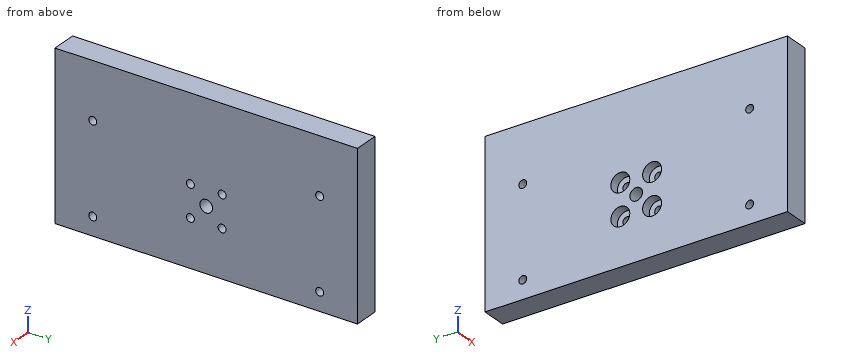
from build123d import *

# Parameters (mm, degrees)
ESQUISSE1_W             = 82.55
ESQUISSE1_H             = 152.4
BOSS_EXTRU_1_DEPTH      = 12.7
ESQUISSE2_R             = 2
ENL_V_MAT_EXTRU_1_DEPTH = 88.586275323
ESQUISSE3_R             = 3.175
ESQUISSE3_R_2           = 2
ENL_V_MAT_EXTRU_2_DEPTH = 88.586275323
ESQUISSE4_R             = 4.7625
ENL_V_MAT_EXTRU_3_DEPTH = 4.7625


with BuildPart() as part:
    # Esquisse1 → Boss.-Extru.1 (new body)
    with BuildSketch(Plane(origin=(0, 0, 0), x_dir=(0, 0, -1), z_dir=(1, 0, 0))):
        Rectangle(ESQUISSE1_W, ESQUISSE1_H)
    extrude(amount=BOSS_EXTRU_1_DEPTH)

    # Esquisse2 → Enlèv. mat.-Extru.1 (cut, through all)
    with BuildSketch(Plane(origin=(12.7, 0, 0), x_dir=(0, 0, -1), z_dir=(1, 0, 0))):
        with Locations((-12.974999958, 57.15)):
            Circle(ESQUISSE2_R)
        with Locations((32.025000042, 57.15)):
            Circle(ESQUISSE2_R)
        with Locations((-12.974999958, -57.15)):
            Circle(ESQUISSE2_R)
        with Locations((32.025000042, -57.15)):
            Circle(ESQUISSE2_R)
    extrude(amount=-ENL_V_MAT_EXTRU_1_DEPTH, mode=Mode.SUBTRACT)

    # Esquisse3 → Enlèv. mat.-Extru.2 (cut, through all)
    with BuildSketch(Plane(origin=(12.7, 0, 0), x_dir=(0, 0, -1), z_dir=(1, 0, 0))):
        with Locations((9.525, 0)):
            Circle(ESQUISSE3_R)
        with Locations((17.525, 8)):
            Circle(ESQUISSE3_R_2)
        with Locations((1.525, 8)):
            Circle(ESQUISSE3_R_2)
        with Locations((1.525, -8)):
            Circle(ESQUISSE3_R_2)
        with Locations((17.525, -8)):
            Circle(ESQUISSE3_R_2)
    extrude(amount=-ENL_V_MAT_EXTRU_2_DEPTH, mode=Mode.SUBTRACT)

    # Esquisse4 → Enlèv. mat.-Extru.3 (cut)
    with BuildSketch(Plane(origin=(0, 0, 0), x_dir=(0, 0, -1), z_dir=(1, 0, 0))):
        with Locations(Location((17.525, 8, 0), (0, 0, 180))):
            Circle(ESQUISSE4_R)
        with Locations(Location((1.525, 8, 0), (0, 0, 180))):
            Circle(ESQUISSE4_R)
        with Locations(Location((1.525, -8, 0), (0, 0, 180))):
            Circle(ESQUISSE4_R)
        with Locations(Location((17.525, -8, 0), (0, 0, 180))):
            Circle(ESQUISSE4_R)
    extrude(amount=ENL_V_MAT_EXTRU_3_DEPTH, mode=Mode.SUBTRACT)


solid = part.part
Build history of the part. All positions in model axes, mm. Coordinates: 2 decimals unless noted, no trailing zeros. Write each loop counter-clockwise with the first axis right and the second up, starting at its lowest first coordinate (ties: lowest second). Pieces come first, ordered by that corner, then holes. Notation, with made-up numbers: (-3.5, 53.25) -> (13.5, 53.25) arc R12 ccw to (13.5, 73.25) -> close; hole circle Ø1 at (70.5, 58). An arc over 180 degrees is marked (long way). Use CSV: the item, a comma, the result in double quotes. Start each with the question number.
Q1. Cut at A-A, the plane y = 8. List the corners of the cut face in (x, z) (1 decimal), then the cut area to 3 significant figures.
Q2. Drill centre lines: probe 1 along Y at (x, z) = (7.5, -31); probe 2 along Z at (x, y) = (1.25, 11) (3 decimals); probe 3 along Z at (x, y) = (7.5, 58) (3 decimals). Where is each one in solid material? Low to high.
Q3. Cut at B-B, the plane x = 3. State how many separate pieces and enclosed holes the cut face has, then the cut area to 3 significant figures.
Q4. Cut at C-C, the plane y = 57.15. List the corners of the cut face in (x, z) (3 decimals), then the cut area to 3 significant figures.
Q5. Flat gauge pins, fed straight in: pin 1 Ø3 at (y, z) = (9, -1.5) entering from -X; pin 2 Ø7.5 at (y, z) = (-8, -17.525) entering from +X. Where does each tip first touch, or does it go through?
Checked values:
1,outline,"(0, -41.3) -> (12.7, -41.3) -> (12.7, -19.5) -> (4.8, -19.5) -> (4.8, -22.3) -> (0, -22.3) -> close; (0, -12.8) -> (4.8, -12.8) -> (4.8, -15.5) -> (12.7, -15.5) -> (12.7, -3.5) -> (4.8, -3.5) -> (4.8, -6.3) -> (0, -6.3) -> close; (0, 3.2) -> (4.8, 3.2) -> (4.8, 0.5) -> (12.7, 0.5) -> (12.7, 41.3) -> (0, 41.3) -> close"
1,area,"894 mm²"
2,probe 1,"y = -76.2 to -58.87, -55.43 to 55.43, 58.87 to 76.2"
2,probe 2,"z = -41.275 to -21.224, -13.826 to -5.224, 2.174 to 41.275"
2,probe 3,"z = -41.275 to -33.835, -30.215 to 11.165, 14.785 to 41.275"
3,separate pieces,"1"
3,enclosed holes,"9"
3,area,"12,200 mm²"
4,outline,"(0, -41.275) -> (12.7, -41.275) -> (12.7, -34.025) -> (0, -34.025) -> close; (0, -30.025) -> (12.7, -30.025) -> (12.7, 10.975) -> (0, 10.975) -> close; (0, 14.975) -> (12.7, 14.975) -> (12.7, 41.275) -> (0, 41.275) -> close"
4,area,"947 mm²"
5,pin 1,"stops at x = 4.76"
5,pin 2,"stops at x = 12.7"
